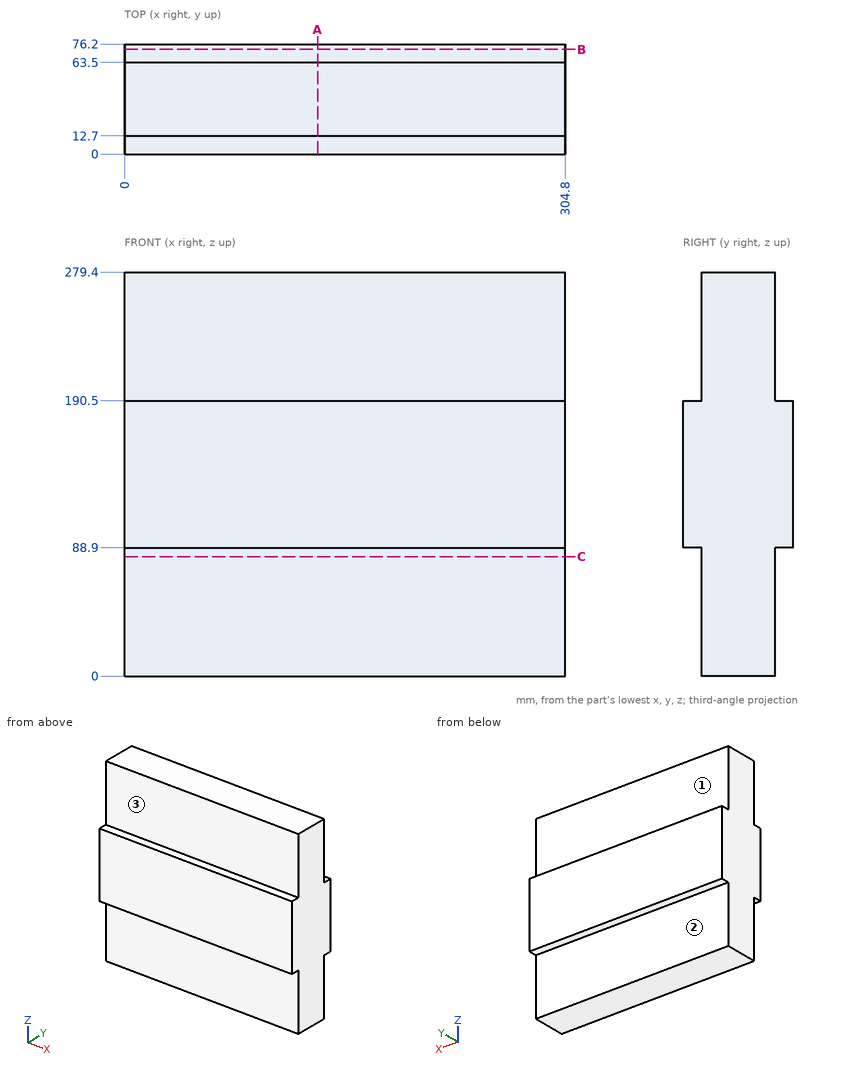
Drawing for the job (mm, zero at the part's lowest x, y, z). A direction names the side the tool comes from. Coordinates: 2 decimals unless noted, no trailing zeros. Loops run counter-clockwise (first coordinate to the right, second up) from the corner with the lowest first, then second, coordinate; pieces in that order, holes last. Notation, with made-up numbers: (37.5, 30) - (56.5, 30) arc R32 cw to (56.5, 63) - close; hole circle Ø2 at (-36, -27.75). An arc over 180 degrees is marked (long way). Return JSON: item names as keys, results as strings.
1. Band-saw the part on C-C (z = 82.5). Give the cut face in (x, y), and give its area (3 significant figures).
Result:
{"outline": "(0, 12.7) - (304.8, 12.7) - (304.8, 63.5) - (0, 63.5) - close", "area": "15,500 mm2"}
2. Probe L1, parallel to Y at x = 120, z = 72.5; L2, parallel to Z at x = 224, y = 10. List the from-to ranges inside material, lowest first. Write a range as from..to.
Result:
{"L1": "y = 12.7..63.5", "L2": "z = 88.9..190.5"}
3. Band-saw the part on B-B (y = 72.5). Give the cut face in (x, z), and give its area (3 significant figures).
Result:
{"outline": "(0, 88.9) - (304.8, 88.9) - (304.8, 190.5) - (0, 190.5) - close", "area": "31,000 mm2"}
4. Drop flat-ended pins along their axis: pin 1 (6.5 mm diameter, centred on x = 186, y = 72.5, fed in from +Z); pin 2 (6.5 mm diameter, centred on x = 174, y = 4, fed in from -Z). Give the stop position or say it passes through.
Result:
{"pin 1": "stops at z = 190.5", "pin 2": "stops at z = 88.9"}
5. 3-axis set-ups, long thin cutter, end or side, ignore diameter. For the marked faces 1, 2 and 3: which of +Z, -Z, +X, -X, +Y, -Y reach the whole face in a straight line?
Result:
{"face 1": "+Z, +X, -X, +Y", "face 2": "-Z, +X, -X, +Y", "face 3": "+Z, +X, -X, -Y"}
6. Band-saw the part on A-A (x = 133.5). Give the cut face in (y, z), and give its area (3 significant figures).
Result:
{"outline": "(0, 88.9) - (12.7, 88.9) - (12.7, 0) - (63.5, 0) - (63.5, 88.9) - (76.2, 88.9) - (76.2, 190.5) - (63.5, 190.5) - (63.5, 279.4) - (12.7, 279.4) - (12.7, 190.5) - (0, 190.5) - close", "area": "16,800 mm2"}
